Geometry: final body of the model. Coordinates: model frame, mm. Face numbers are marked on the shaded views. Give positions to 0.01 mm unless a question says otherwise; leave off trailing zeros. Loops run counter-clockwise (first coordinate to the right, second up) from the corner with the lowest first, then second, coordinate; pieces in that order, holes last. Notation, with made-up numbers: (89, 34.25) - (100, 34.25) arc R14 ccw to (100, 51.25) - close; hole circle Ø8 at (-21, 60.25). An arc over 180 degrees is marked (long way). Use one line per item in the form item = value.
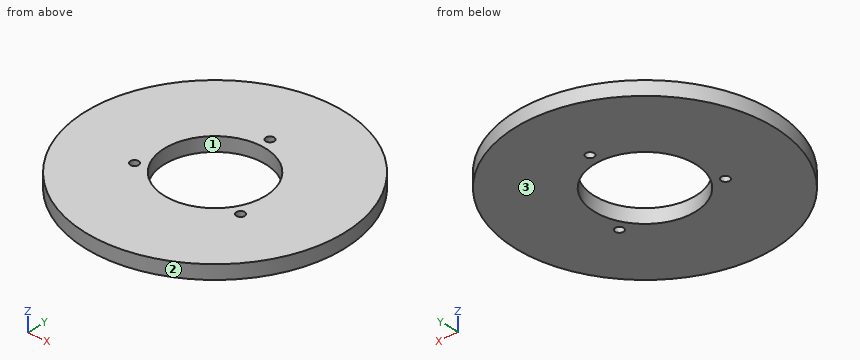
```python
from build123d import *

# Parameters (mm, degrees)
SKETCH2_R               = 46
SKETCH2_R_2             = 18
BOSS_EXTRUDE2_DEPTH     = 5
SKETCH5_R               = 1.5
CUT_EXTRUDE1_DEPTH      = 1
CUT_EXTRUDE1_DEPTH_BACK = 6


with BuildPart() as part:
    # Sketch2 → Boss-Extrude2 (new body)
    with BuildSketch(Plane.XY):
        Circle(SKETCH2_R)
        Circle(SKETCH2_R_2, mode=Mode.SUBTRACT)
    extrude(amount=BOSS_EXTRUDE2_DEPTH)

    # Sketch5 → Cut-Extrude1 (cut, two sides)
    with BuildSketch(Plane(origin=(0, 0, 0), x_dir=(-1, 0, 0), z_dir=(0, 0, -1))) as cut_extrude1_sk:
        with Locations((0, 22)):
            Circle(SKETCH5_R)
        with Locations((19.052558883, -11)):
            Circle(SKETCH5_R)
        with Locations((-19.052558883, -11)):
            Circle(SKETCH5_R)
    extrude(amount=CUT_EXTRUDE1_DEPTH, mode=Mode.SUBTRACT)
    extrude(cut_extrude1_sk.sketch, amount=-CUT_EXTRUDE1_DEPTH_BACK, mode=Mode.SUBTRACT)


solid = part.part
```
(1) Cut plane D-D (x = 13). Return the cut outline in (y, z).
Solution:
outline = (-44.12, 0) - (-12.45, 0) - (-12.45, 5) - (-44.12, 5) - close; (12.45, 0) - (44.12, 0) - (44.12, 5) - (12.45, 5) - close
(2) Cut plane C-C (z = 2.05). Return the cut outline in (x, y), plus the area to 3 significant figures.
Solution:
outline = circle Ø92 at (0, 0); hole circle Ø3 at (-19.05, -11); hole circle Ø36 at (0, 0); hole circle Ø3 at (0, 22); hole circle Ø3 at (19.05, -11)
area = 5,610 mm2
(3) Cut plane A-A (y = 0). Return the cut outline in (x, z), plus the area to 3 significant figures.
Solution:
outline = (-46, 0) - (-18, 0) - (-18, 5) - (-46, 5) - close; (18, 0) - (46, 0) - (46, 5) - (18, 5) - close
area = 280 mm2
(4) Cut plane B-B (x = 0). Return the cut outline in (y, z), plus the area to 3 significant figures.
Solution:
outline = (-46, 0) - (-18, 0) - (-18, 5) - (-46, 5) - close; (18, 0) - (20.5, 0) - (20.5, 5) - (18, 5) - close; (23.5, 0) - (46, 0) - (46, 5) - (23.5, 5) - close
area = 265 mm2
(5) Pin query (flat end, axial travel): P1, Ø1, axis at x = 11, z = 2, coming from the +Y side; P2, Ø2, axis at y = 26.5, z = 2, coming from the +X side; P3, Ø2, axis at x = -36.5, z = 3.5, coming from the +Y side; P4, Ø2.5, axis at x = 19.05, y = -11, coming from the +Z side. Return the tip coordinate at first contact, or that it passes through.
Solution:
P1 = 44.79
P2 = 38.29
P3 = 29.25
P4 = through
(6) Pull-direction query (Y, two-part tool) for the marked faces 1, 2 and 3; classes: released by +Y, released by -Y, zero draft, split by the parting line, or undercut.
Solution:
face_1 = undercut
face_2 = split by the parting line
face_3 = zero draft
(7) Material intervals for L1, parallel to Y at x = 0, z = 2.85; L2, parallel to Y at x = 1, z = 0.5; L3, parallel to X at y = -10, z = 2.85, sorted ascending. Write a range as from..to.
Solution:
L1 = -46..-18, 18..20.5, 23.5..46
L2 = -45.99..-17.97, 17.97..20.88, 23.12..45.99
L3 = -44.9..-20.17, -17.93..-14.97, 14.97..17.93, 20.17..44.9
